For this review, take the finished solid that the model builds, in its own axes (mm). Face numbers are marked on the shaded views. Coordinates: 2 decimals unless noted, no trailing zeros. Write each loop counter-clockwise with the first axis right and the second up, starting at its lowest first coordinate (ties: lowest second). Pieces come first, ordered by that corner, then holes. Notation, with made-up numbers: (28.25, 37) - (52.25, 37) arc R25 ccw to (52.25, 53) - close; hole circle Ø3 at (-22.5, -25.75). An arc over 180 degrees is marked (long way). Write each question's results on one line, items separated by ' | '.
from build123d import *
from build123d.topology import SkipClean

# Parameters (mm, degrees)
SKETCH2_R                = 56.515
SKETCH2_R_2              = 51.435
BOSS_EXTRUDE1_DEPTH      = 35
SKETCH2_R_3              = 47.201666667
SKETCH2_R_4              = 42.121666667
BOSS_EXTRUDE1_2_DEPTH    = 35
SKETCH3_R                = 56.515
BOSS_EXTRUDE2_DEPTH      = 15.24
CUT_EXTRUDE1_DEPTH       = 95.40311462
CUT_EXTRUDE1_DEPTH_BACK  = 95.40311462
SKETCH4_R                = 1.6
SKETCH4_R_2              = 1.65876763
SKETCH4_R_3              = 1.651
CUT_EXTRUDE18_REACH      = 96.403
SKETCH32_R               = 2.6
SKETCH_1_R               = 6
CUT_EXTRUDE_1_DEPTH      = 5
CUT_EXTRUDE_2_REACH      = 137.992
CUT_EXTRUDE_2_END_RADIUS = 42.121666667
SKETCH_3_R               = 10
SKETCH_4_R               = 15
SKETCH_4_R_2             = 10
EXTRUDE_1_DEPTH          = 17.154678362
SKETCH_10_W              = 5
SKETCH_10_H              = 4.233333333
SKETCH_10_H_2            = 4.444320869
EXTRUDE_3_DEPTH          = 33
CUT_EXTRUDE_START        = -40
SKETCH_11_R              = 61.515
SKETCH_11_R_2            = 56.515
CUT_EXTRUDE_3_DEPTH      = 30
SKETCH_15_W              = 2.458765136
SKETCH_15_H              = 28
EXTRUDE_9_DEPTH          = 5


with BuildPart() as part:
    # Sketch2 → Boss-Extrude1 (new body)
    with BuildSketch(Plane(origin=(0, 0, 0), x_dir=(1, 0, 0), z_dir=(0, 1, 0))):
        with Locations(Location((0, 0, 0), (0, 0, 270))):
            Circle(SKETCH2_R)
        with Locations(Location((0, 0, 0), (0, 0, 270))):
            Circle(SKETCH2_R_2, mode=Mode.SUBTRACT)
    extrude(amount=BOSS_EXTRUDE1_DEPTH)



with BuildPart() as body_2:
    # Sketch2 → Boss-Extrude1 2 (new body)
    with BuildSketch(Plane(origin=(0, 0, 0), x_dir=(1, 0, 0), z_dir=(0, 1, 0))):
        with Locations(Location((0, 0, 0), (0, 0, 270))):
            Circle(SKETCH2_R_3)
        with Locations(Location((0, 0, 0), (0, 0, 270))):
            Circle(SKETCH2_R_4, mode=Mode.SUBTRACT)
    extrude(amount=BOSS_EXTRUDE1_2_DEPTH)


with BuildPart() as part_1:
    add(part.part)

    add(body_2.part)  # Boss-Extrude2 merges body 2
    # Sketch3 → Boss-Extrude2 (add)
    with BuildSketch(Plane(origin=(0, 35, 0), x_dir=(1, 0, 0), z_dir=(0, 1, 0))):
        with Locations(Location((0, 0, 0), (0, 0, 270))):
            Circle(SKETCH3_R)
    extrude(amount=BOSS_EXTRUDE2_DEPTH)

    # Sketch4 → Cut-Extrude1 (cut, two sides: drawn at the far end of the back side and taken through both)
    with BuildSketch(Plane(origin=(0, 50.24, 0), x_dir=(1, 0, 0), z_dir=(0, 1, 0)).offset(-CUT_EXTRUDE1_DEPTH_BACK)):
        with Locations(Location((20.859650045, 20.859650045, 0), (0, 0, 270))):
            Circle(SKETCH4_R)
        with Locations(Location((20.859650045, -20.859650045, 0), (0, 0, 270))):
            Circle(SKETCH4_R)
        with Locations(Location((-20.859650045, -20.859650045, 0), (0, 0, 270))):
            Circle(SKETCH4_R_2)
        with Locations(Location((-20.859650045, 20.859650045, 0), (0, 0, 270))):
            Circle(SKETCH4_R_3)
    extrude(amount=CUT_EXTRUDE1_DEPTH + CUT_EXTRUDE1_DEPTH_BACK, mode=Mode.SUBTRACT)

    # Sketch32 → Cut-Extrude18 (cut, up to next)
    with BuildSketch(Plane(origin=(0, 50.24, 0), x_dir=(1, 0, 0), z_dir=(0, 1, 0)), mode=Mode.PRIVATE) as cut_extrude18_sk1:
        with Locations(Location((30, 11.5, 0), (0, 0, 270))):
            Circle(SKETCH32_R)
    cut_extrude18_tool1 = extrude(cut_extrude18_sk1.sketch, amount=-CUT_EXTRUDE18_REACH, mode=Mode.PRIVATE) & part_1.part
    # Sketch32 → Cut-Extrude18 (cut, up to next)
    with BuildSketch(Plane(origin=(0, 50.24, 0), x_dir=(1, 0, 0), z_dir=(0, 1, 0)), mode=Mode.PRIVATE) as cut_extrude18_sk2:
        with Locations(Location((30, -11.5, 0), (0, 0, 270))):
            Circle(SKETCH32_R)
    cut_extrude18_tool2 = extrude(cut_extrude18_sk2.sketch, amount=-CUT_EXTRUDE18_REACH, mode=Mode.PRIVATE) & part_1.part
    # Sketch32 → Cut-Extrude18 (cut, up to next)
    with BuildSketch(Plane(origin=(0, 50.24, 0), x_dir=(1, 0, 0), z_dir=(0, 1, 0)), mode=Mode.PRIVATE) as cut_extrude18_sk3:
        with Locations(Location((-30, -11.5, 0), (0, 0, 270))):
            Circle(SKETCH32_R)
    cut_extrude18_tool3 = extrude(cut_extrude18_sk3.sketch, amount=-CUT_EXTRUDE18_REACH, mode=Mode.PRIVATE) & part_1.part
    # Sketch32 → Cut-Extrude18 (cut, up to next)
    with BuildSketch(Plane(origin=(0, 50.24, 0), x_dir=(1, 0, 0), z_dir=(0, 1, 0)), mode=Mode.PRIVATE) as cut_extrude18_sk4:
        with Locations(Location((-30, 11.5, 0), (0, 0, 270))):
            Circle(SKETCH32_R)
    cut_extrude18_tool4 = extrude(cut_extrude18_sk4.sketch, amount=-CUT_EXTRUDE18_REACH, mode=Mode.PRIVATE) & part_1.part
    add(cut_extrude18_tool1.solids().sort_by_distance((30, 50.24, -11.5))[0], mode=Mode.SUBTRACT)
    add(cut_extrude18_tool2.solids().sort_by_distance((30, 50.24, 11.5))[0], mode=Mode.SUBTRACT)
    add(cut_extrude18_tool3.solids().sort_by_distance((-30, 50.24, 11.5))[0], mode=Mode.SUBTRACT)
    add(cut_extrude18_tool4.solids().sort_by_distance((-30, 50.24, -11.5))[0], mode=Mode.SUBTRACT)

    # 草图1 → 切除-拉伸1 (cut)
    with BuildSketch(Plane(origin=(0, 35, 0), x_dir=(-1, 0, 0), z_dir=(0, -1, 0))):
        with Locations(Location((30, 11.5, 0), (0, 0, 90))):
            Circle(SKETCH_1_R)
        with Locations(Location((30, -11.5, 0), (0, 0, 90))):
            Circle(SKETCH_1_R)
        with Locations(Location((-30, 11.5, 0), (0, 0, 90))):
            Circle(SKETCH_1_R)
        with Locations(Location((-30, -11.5, 0), (0, 0, 90))):
            Circle(SKETCH_1_R)
    extrude(amount=-CUT_EXTRUDE_1_DEPTH, mode=Mode.SUBTRACT)

    # 切除-拉伸2: up to this cylinder (the profile starts outside it)
    cut_extrude_2_end = Plane(origin=(0, 25, 0), z_dir=(0, -1, 0)) * Cylinder(CUT_EXTRUDE_2_END_RADIUS, 361.227333333, mode=Mode.PRIVATE)
    # 草图3 → 切除-拉伸2 (cut, up to the surface)
    with BuildSketch(Plane.XY.offset(-56.515), mode=Mode.PRIVATE) as cut_extrude_2_sk1:
        with Locations(Location((0, 25, 0), (0, 0, 270))):
            Circle(SKETCH_3_R)
    cut_extrude_2_tool1 = extrude(cut_extrude_2_sk1.sketch, amount=CUT_EXTRUDE_2_REACH, mode=Mode.PRIVATE) - cut_extrude_2_end
    add(cut_extrude_2_tool1.solids().sort_by_distance((0, 25, -56.515))[0], mode=Mode.SUBTRACT)

    # 草图4 → 拉伸-薄壁1 (add)
    with SkipClean():  # the faces are left unmerged after this step: merging them gives an invalid solid
        with BuildSketch(Plane.XY.offset(-56.515)):
            with Locations((0, 25)):
                Circle(SKETCH_4_R)
            with Locations((0, 25)):
                Circle(SKETCH_4_R_2, mode=Mode.SUBTRACT)
        extrude(amount=EXTRUDE_1_DEPTH)

    # 草图10 → 拉伸-薄壁3 (add)
    with SkipClean():  # the faces are left unmerged after this step: merging them gives an invalid solid
        with BuildSketch(Plane(origin=(0, 7, 0), x_dir=(1, 0, 0), z_dir=(0, 1, 0))):
            with Locations((2.5, 49.318333334)):
                Rectangle(SKETCH_10_W, SKETCH_10_H)
            with Locations((-12.5, 46.977018675)):
                Rectangle(SKETCH_10_W, SKETCH_10_H_2)
            with Locations((17.5, 46.977018675)):
                Rectangle(SKETCH_10_W, SKETCH_10_H_2)
            with BuildLine():
                ThreePointArc((15.089267159, 49.171874498), (0, 51.435), (-15.089267159, 49.171874498))
                Line((-15.089267159, 49.171874498), (-16.55609589, 53.951875907))
                ThreePointArc((-16.55609589, 53.951875907), (0, 56.435), (16.55609589, 53.951875907))
                Line((16.55609589, 53.951875907), (15.089267159, 49.171874498))
            make_face()
            with BuildLine():
                ThreePointArc((15.111664358, 44.717277829), (0, 47.201666667), (-15.111664358, 44.717277829))
                Line((-15.111664358, 44.717277829), (-16.712419736, 49.454110338))
                ThreePointArc((-16.712419736, 49.454110338), (0, 52.201666667), (16.712419736, 49.454110338))
                Line((16.712419736, 49.454110338), (15.111664358, 44.717277829))
            make_face()
        extrude(amount=EXTRUDE_3_DEPTH)

    # 草图11 → 切除-拉伸-薄壁3 (cut)
    with SkipClean():  # the faces are left unmerged after this step: merging them gives an invalid solid
        with BuildSketch(Plane(origin=(0, 0, 0), x_dir=(-1, 0, 0), z_dir=(0, -1, 0)).offset(CUT_EXTRUDE_START)):
            Circle(SKETCH_11_R)
            Circle(SKETCH_11_R_2, mode=Mode.SUBTRACT)
        extrude(amount=CUT_EXTRUDE_3_DEPTH, mode=Mode.SUBTRACT)

    # 草图15 → 凸台-拉伸9 (add)
    with BuildSketch(Plane(origin=(20, 0, 0), x_dir=(0, 0, -1), z_dir=(1, 0, 0))):
        with Locations((43.525475672, 21)):
            Rectangle(SKETCH_15_W, SKETCH_15_H)
    extrude(amount=-EXTRUDE_9_DEPTH)


solid = part_1.part
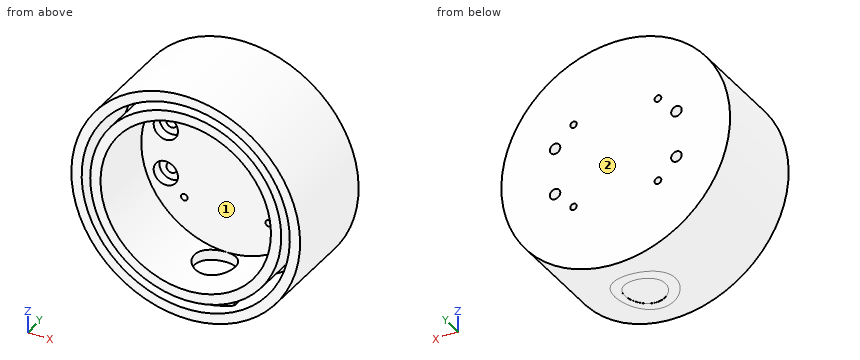
Q1. Wall thickness on line 1 along Z through (x, y) = (0, 24.5) (3 decimals); line 2 along X through (y, z) = (23.5, -2); line 3 along Z through (x, y) = (18.5, 2.5): over which ranges is each line inside the solid? List them lowest first. Write a range as from..to.
Results found:
line 1: -56.435..-47.202, 42.122..47.202, 51.435..56.515 | line 2: -56.48..-51.4, -47.16..-42.07, 42.07..47.16, 51.4..56.48 | line 3: -53.4..-47.99, -43.43..-37.84, 37.84..43.43, 47.99..53.4
Q2. For pin 1 (1 mm diameter, centred on x = 37.5, y = 43, fed in from -Z); pin 2 (10 mm diameter, centred on y = 37, z = 18.5, fed in from -X); pin 3 (5 mm diameter, centred on x = -14, y = 5.5, fed in from -Z), all flat-tipped, find the tip position at first contact; note any pin that passes through.
Results found:
pin 1: z = -42.72 | pin 2: x = -54.88 | pin 3: z = -55.33
Q3. Mouldability with a two-part tool opening along X and no side actions: class the marked faces 1 and 2 as pulls with the +X half, pulls with the -X half, needs draft (parallel to the pull), parting line crosses it, or undercut.
Results found:
face 1: undercut | face 2: needs draft
Q4. Take a section at D-D on y = 17. State the section outline as (x, z) points (3 decimals).
Results found:
outline: (-6, -56.196) - (-6, -56.115) arc R56.435 ccw to (6, -56.115) - (6, -56.196) arc R56.515 ccw (long way) to start; hole (-16.467, -48.728) - (-15.112, -44.717) arc R47.202 cw (long way) to (20, -42.755) - (20, -47.387) arc R51.435 ccw (long way) to start; hole (-6, -46.819) arc R47.202 ccw to (6, -46.819) - (6, -41.692) arc R42.122 ccw (long way) to (-6, -41.692) - close
Q5. Take a section at A-A on z = 11.5. State how many separate pieces and enclosed holes the cut face has, plus the area to 3 significant figures.
Results found:
separate pieces: 3 | enclosed holes: 0 | area: 2,190 mm2
